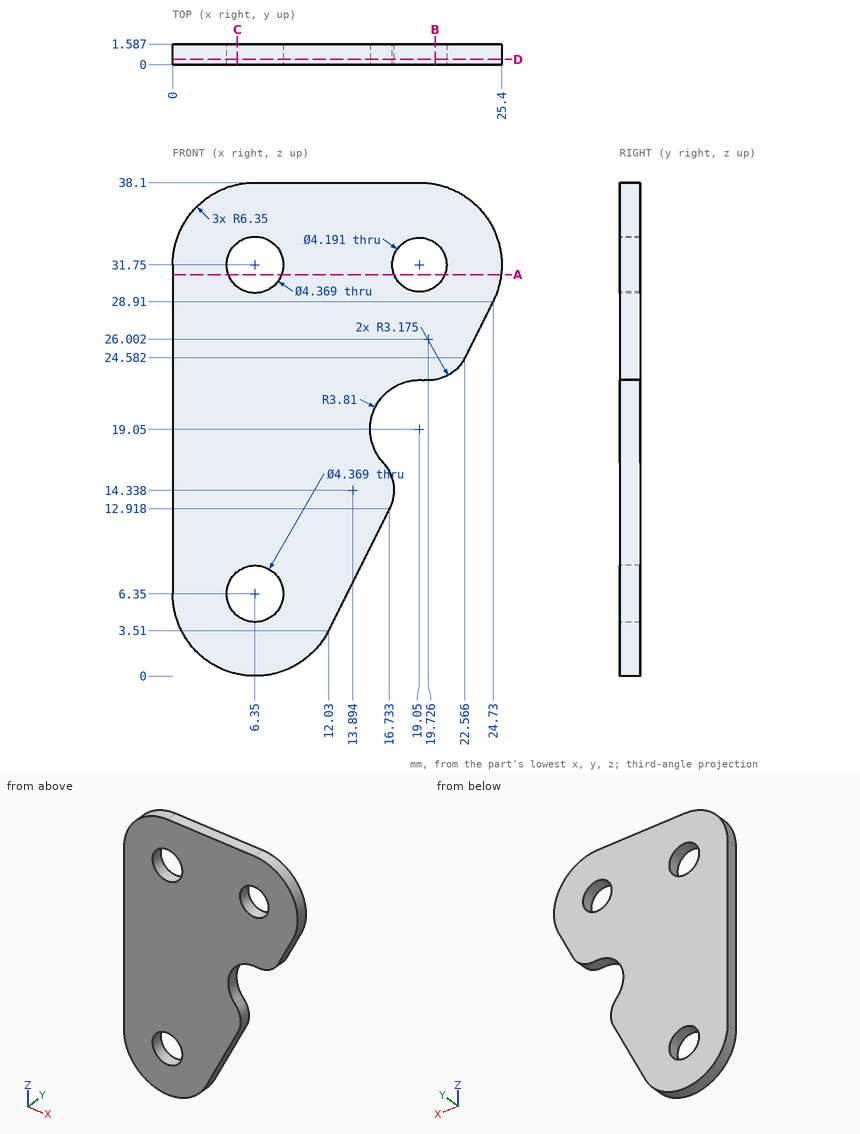
Job drawing, mm, ordinate dimensions from the low corner. One solid piece. Give positions to 0.01 mm unless a question says otherwise; leave off trailing zeros. Order: outer loops, then holes, each group sorted by start corner. A loop starts at its lowest first (then second) coordinate and runs counter-clockwise, first axis right, second up. Notation, with made-up numbers: M 10,59 L 26,59 A20 cw 26,98 Z; hole C -10,61.5 d3. An arc over 180 degrees is marked long. Put each result on its own line as item: value. Start each with the question number.
(1) Band-saw the part on D-D on y = 0.4. Count the separate pieces of the cut face and the enclosed holes in it, then the cut area to 3 significant figures.
(2) Band-saw the part on C-C on x = 5. Give the cut face in (y, z) (1 decimal).
(3) Pin check, flat tips, straight feed: pin 1 Ø7 at (x, z) = (6.35, 31.75) entering from -Y; pin 2 Ø3.5 at (x, z) = (6.35, 6.35) entering from -Y. Stop position of each tip, or through.
(4) Band-saw the part on A-A on z = 31. Give the cut face in (x, y) (1 decimal).
(5) Band-saw the part on B-B on x = 20.25. Give the cut face in (y, z) (1 decimal).
(6) Drill centre lines: L1, parallel to Z at x = 6.35, y = 0.9 (1 decimal); L2, parallel to Z at x = 19.05, y = 0.95 (1 decimal); L3, parallel to X at y = 0.45, z = 32.5 (1 decimal). Where is each one in solid material? Low to high. Write a range as [from, to].
Results below:
1. separate pieces: 1
1. enclosed holes: 3
1. area: 636 mm2
2. outline: M 0,0.1 L 1.6,0.1 L 1.6,4.6 L 0,4.6 Z; M 0,8.1 L 1.6,8.1 L 1.6,30 L 0,30 Z; M 0,33.5 L 1.6,33.5 L 1.6,38 L 0,38 Z
3. pin 1: stops at y = 0
3. pin 2: passes through
4. outline: M 0,0 L 4.3,0 L 4.3,1.6 L 0,1.6 Z; M 8.4,0 L 17.1,0 L 17.1,1.6 L 8.4,1.6 Z; M 21,0 L 25.4,0 L 25.4,1.6 L 21,1.6 Z
5. outline: M 0,22.9 L 1.6,22.9 L 1.6,30 L 0,30 Z; M 0,33.5 L 1.6,33.5 L 1.6,38 L 0,38 Z
6. L1: z = [0, 4.2], [8.5, 29.6], [33.9, 38.1]
6. L2: z = [22.9, 29.7], [33.8, 38.1]
6. L3: x = [0, 4.3], [8.4, 17.1], [21, 25.4]
